```python
from build123d import *

# Parameters (mm, degrees)
SZKIC1_W                       = 237
SZKIC1_H                       = 197
DODANIE_WYCI_GNI_CIE1_DEPTH    = 2.5
SZKIC2_W                       = 29
SZKIC2_H                       = 35
WYTNIJ_WYCI_GNI_CIE1_DEPTH     = 3
SZYK_LINIOWY1_COUNT            = 3
SZYK_LINIOWY1_PITCH            = 75
OTWORY_USTALAJ_CE_4_0MM1_D     = 3.5
OTWORY_USTALAJ_CE_4_0MM1_DEPTH = 10


with BuildPart() as part:
    # Szkic1 → Dodanie-wyciągnięcie1 (new body)
    with BuildSketch(Plane(origin=(0, 0, 0), x_dir=(1, 0, 0), z_dir=(0, 1, 0))):
        with Locations((118.5, 98.5)):
            Rectangle(SZKIC1_W, SZKIC1_H)
    extrude(amount=DODANIE_WYCI_GNI_CIE1_DEPTH)

    # Szkic2 → Wytnij-wyciągnięcie1 (cut)
    with BuildSketch(Plane(origin=(0, 2.5, 0), x_dir=(1, 0, 0), z_dir=(0, 1, 0))):
        with Locations((30.5, 17.5)):
            Rectangle(SZKIC2_W, SZKIC2_H)
    wytnij_wyci_gni_cie1 = extrude(amount=-WYTNIJ_WYCI_GNI_CIE1_DEPTH, mode=Mode.SUBTRACT)

    # Szyk liniowy1: Wytnij-wyciągnięcie1 ×3
    with Locations(*[(i * SZYK_LINIOWY1_PITCH, 0, 0) for i in range(1, SZYK_LINIOWY1_COUNT)]):
        add(wytnij_wyci_gni_cie1, mode=Mode.SUBTRACT)

    # Otwory ustalające Ø4.0mm1
    with Locations(Plane(origin=(0, 2.5, 0), x_dir=(1, 0, 0), z_dir=(0, 1, 0))):
        with Locations((6.5, 6), (53, 6), (84, 6), (84, 98.280811552), (6.5, 97.43634097), (6.5, 188.669995221), (52.411150371, 189), (84, 189), (127.411150371, 189), (128, 6), (159, 6), (203, 6), (234, 6), (159, 98.280811552), (234, 98.280811552), (234, 189), (202.411150371, 189), (159, 189), (6.5, 40), (84, 40), (159, 40), (234, 40)):
            Hole(OTWORY_USTALAJ_CE_4_0MM1_D / 2, depth=OTWORY_USTALAJ_CE_4_0MM1_DEPTH)


solid = part.part
```
Part model, mm, in its own coordinate system. Coordinates: 2 decimals unless noted, no trailing zeros. Order: outer loops, then holes, each group sorted by start corner. A loop starts at its lowest first (then second) coordinate and runs counter-clockwise, first axis right, second up. Notation, with made-up numbers: (27.5, 68) - (52.5, 68) arc R22 cw to (52.5, 98) - close; hole circle Ø1 at (-26, -11). An arc over 180 degrees is marked (long way). Return JSON: item names as keys, results as strings. Group by question number.
Item 1: Cut at C-C (y = 1.9). State how many separate pieces and enclosed holes the cut face has, plus the area to 3 significant figures.
Item 2: Cut at A-A (z = -24). List the corners of the cut face in (x, y), plus the area to 3 significant figures.
Item 3: Pin check, flat tip, straight feed: pin 1 (0.8 mm diameter, centred on x = 36.5, y = 2, fed in from +Z). Stop position of the tip, or through.
Item 4: Cut at B-B (x = 172.5). List the corners of the cut face in (y, z), plus the area to 3 significant figures.
Item 5: Drill centre lines: probe 1 along X at (y, z) = (0.85, -40); probe 2 along X at (y, z) = (2.35, -17); probe 3 along Z at (x, y) = (6.5, 1.3). Where is each one in solid material? Low to high. Write a range as from..to.
Check values:
{
 "1": {"separate pieces": "1", "enclosed holes": "22", "area": "43,400 mm2"},
 "2": {"outline": "(0, 0) - (16, 0) - (16, 2.5) - (0, 2.5) - close; (45, 0) - (91, 0) - (91, 2.5) - (45, 2.5) - close; (120, 0) - (166, 0) - (166, 2.5) - (120, 2.5) - close; (195, 0) - (237, 0) - (237, 2.5) - (195, 2.5) - close", "area": "375 mm2"},
 "3": {"pin 1": "stops at z = -35"},
 "4": {"outline": "(0, -197) - (2.5, -197) - (2.5, -35) - (0, -35) - close", "area": "405 mm2"},
 "5": {"probe 1": "x = 0..4.75, 8.25..82.25, 85.75..157.25, 160.75..232.25, 235.75..237", "probe 2": "x = 0..16, 45..91, 120..166, 195..237", "probe 3": "z = -197..-190.42, -186.92..-99.19, -95.69..-41.75, -38.25..-7.75, -4.25..0"}
}
